Geometry check sheet. Reference: drawing and pictorial views, mm from the part's lowest x, y, z. A direction names the side the tool comes from. Give positions to 0.01 mm unless a question says otherwise; leave off trailing zeros. Write each loop counter-clockwise with the first axis right and the second up, starting at its lowest first coordinate (ties: lowest second). Pieces come first, ordered by that corner, then holes. Notation, with made-up numbers: (16, -20.75) - (61, -20.75) arc R17 cw to (61, -1.75) - close; hole circle Ø7 at (10, 20). An arc over 180 degrees is marked (long way). Put each result on its own line as item: value.
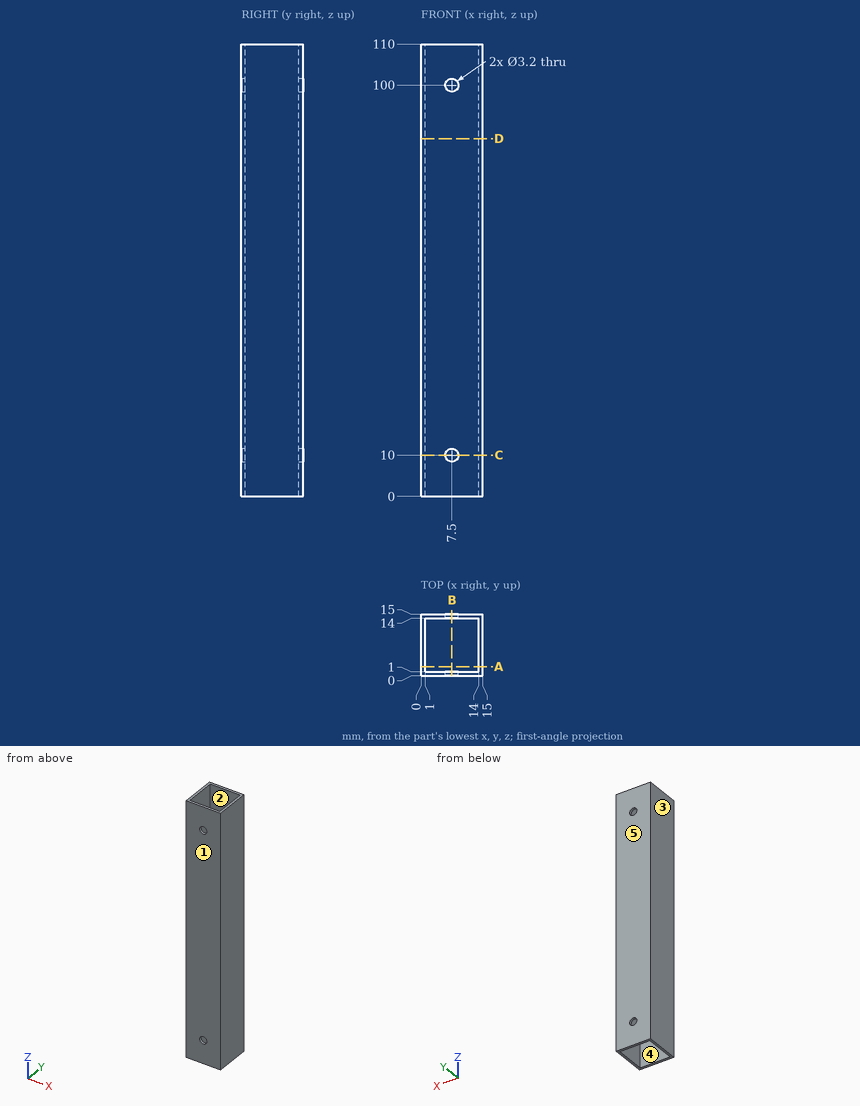
Q1. Set-up check for the marked faces 1 and 2: record each of +Z, -Z, +X, -X, +Y, -Y from which the full face is reachable in a straight line by a thin tool's end or side.
Answers follow:
face 1: +Z, -Z, +X, -X, -Y
face 2: +Z, -Z
Q2. Release check for a two-part mould opening along Y. For the marked faces 3, 4 and 5 record: released by +Y, released by -Y, zero draft, split by the parting line, or undercut.
Answers follow:
face 3: zero draft
face 4: undercut
face 5: released by +Y
Q3. Scan lines: line 1 along Y through (x, z) = (6, 94); line 2 along X through (y, z) = (0.55, 100). Record each from-to range of solid material in increasing order.
Answers follow:
line 1: y = 0 to 1, 14 to 15
line 2: x = 0 to 5.9, 9.1 to 15
Q4. Section check C-C, the plane z = 10. Record the cut outline in (x, y), plus the area to 3 significant figures.
Answers follow:
outline: (0, 0) - (5.9, 0) - (5.9, 1) - (1, 1) - (1, 14) - (5.9, 14) - (5.9, 15) - (0, 15) - close; (9.1, 0) - (15, 0) - (15, 15) - (9.1, 15) - (9.1, 14) - (14, 14) - (14, 1) - (9.1, 1) - close
area: 49.6 mm2
Q5. Section check A-A, the plane y = 2.25. Record the cut outline in (x, z), plus the area to 3 significant figures.
Answers follow:
outline: (0, 0) - (1, 0) - (1, 110) - (0, 110) - close; (14, 0) - (15, 0) - (15, 110) - (14, 110) - close
area: 220 mm2
Q6. Go/stop test with a flat-tipped pin: pin 1 Ø8 at (x, z) = (7, 85) entering from -Y. Record where the tip stops, or that it passes through.
Answers follow:
pin 1: stops at y = 0
Q7. Section check D-D, the plane z = 87. Record the cut outline in (x, y).
Answers follow:
outline: (0, 0) - (15, 0) - (15, 15) - (0, 15) - close; hole (1, 1) - (14, 1) - (14, 14) - (1, 14) - close
Q8. Section check B-B, the plane x = 7.5. Record the cut outline in (y, z), plus the area to 3 significant figures.
Answers follow:
outline: (0, 0) - (1, 0) - (1, 8.4) - (0, 8.4) - close; (0, 11.6) - (1, 11.6) - (1, 98.4) - (0, 98.4) - close; (0, 101.6) - (1, 101.6) - (1, 110) - (0, 110) - close; (14, 0) - (15, 0) - (15, 8.4) - (14, 8.4) - close; (14, 11.6) - (15, 11.6) - (15, 98.4) - (14, 98.4) - close; (14, 101.6) - (15, 101.6) - (15, 110) - (14, 110) - close
area: 207 mm2
